The drawing under review shows one solid part. Ordinate dimensions are in mm from its lowest x, y, z. A direction names the side the tool comes from. Give positions to 0.01 mm unless a question says otherwise; leave off trailing zeros. Write each loop counter-clockwise with the first axis right and the second up, starting at its lowest first coordinate (ties: lowest second). Pieces come first, ordered by that corner, then holes. Notation, with made-up numbers: (-7.5, 2) -> (15.5, 2) arc R26 ccw to (15.5, 38) -> close; hole circle Ø4 at (71.25, -35). An arc over 180 degrees is marked (long way). Answer as a JSON object with one key per item and string values.
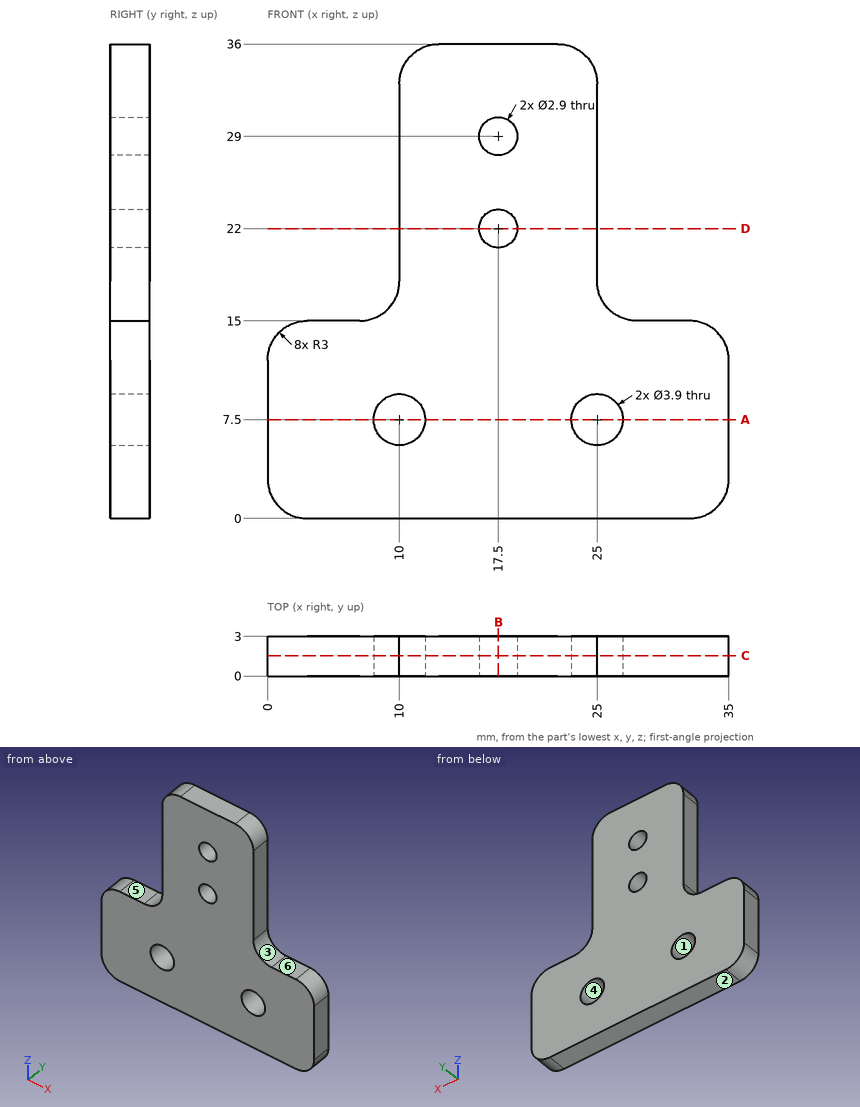
(1) We need section B-B, the plane x = 17.5. State the section outline as (y, z) points.
Here are the results:
{"outline": "(0, 0) -> (3, 0) -> (3, 20.55) -> (0, 20.55) -> close; (0, 23.45) -> (3, 23.45) -> (3, 27.55) -> (0, 27.55) -> close; (0, 30.45) -> (3, 30.45) -> (3, 36) -> (0, 36) -> close"}
(2) Clearance check with flat-ended pins moving along their axes: pin 1 (1.5 mm diameter, centred on x = 30.5, y = 1.5, fed in from +Z); pin 2 (1.5 mm diameter, centred on y = 1, z = 22, fed in from -X); pin 3 (0.9 mm diameter, centred on y = 2, z = 28, fed in from +X); pin 4 (2.5 mm diameter, centred on x = 17.5, z = 22, fed in from -Y). State where each tip first meets the part, or that it passes through.
Here are the results:
{"pin 1": "stops at z = 15", "pin 2": "stops at x = 10", "pin 3": "stops at x = 25", "pin 4": "passes through"}
(3) We need section A-A, the plane z = 7.5. State the section outline as (x, y) points.
Here are the results:
{"outline": "(0, 0) -> (8.05, 0) -> (8.05, 3) -> (0, 3) -> close; (11.95, 0) -> (23.05, 0) -> (23.05, 3) -> (11.95, 3) -> close; (26.95, 0) -> (35, 0) -> (35, 3) -> (26.95, 3) -> close"}
(4) For the marked faces 4, 5 and 6, list the 3-axis set-ups (+Z, -Z, +X, -X, +Y, -Y) from which the entire face can be reached by the end or side of a thin tool; tool diameter is ignored.
Here are the results:
{"face 4": "+Y, -Y", "face 5": "+Z, -X, +Y, -Y", "face 6": "+Z, +X, +Y, -Y"}
(5) The part is to be moulded in two halves that separate along Z. For the marked faces 1, 2 and 3, say which applies: +Z half, -Z half, draft (parallel to the pull), parting line (faces both ways), or undercut.
Here are the results:
{"face 1": "undercut", "face 2": "-Z half", "face 3": "+Z half"}
(6) For line 1 along X through (y, z) = (2.45, 7.5); line 2 along X through (y, z) = (1.85, 29); line 3 along X through (y, z) = (1.6, 30.5), list the stretches that pass through material, from the lowest coordinate up.
Here are the results:
{"line 1": "x = 0 to 8.05, 11.95 to 23.05, 26.95 to 35", "line 2": "x = 10 to 16.05, 18.95 to 25", "line 3": "x = 10 to 25"}
(7) We need section D-D, the plane z = 22. State the section outline as (x, y) points, then the cut area to 3 significant figures.
Here are the results:
{"outline": "(10, 0) -> (16.05, 0) -> (16.05, 3) -> (10, 3) -> close; (18.95, 0) -> (25, 0) -> (25, 3) -> (18.95, 3) -> close", "area": "36.3 mm²"}
(8) We need section C-C, the plane y = 1.55. State the section outline as (x, z) points, then the cut area to 3 significant figures.
Here are the results:
{"outline": "(0, 3) arc R3 ccw to (3, 0) -> (32, 0) arc R3 ccw to (35, 3) -> (35, 12) arc R3 ccw to (32, 15) -> (28, 15) arc R3 cw to (25, 18) -> (25, 33) arc R3 ccw to (22, 36) -> (13, 36) arc R3 ccw to (10, 33) -> (10, 18) arc R3 cw to (7, 15) -> (3, 15) arc R3 ccw to (0, 12) -> close; hole circle Ø3.9 at (10, 7.5); hole circle Ø2.9 at (17.5, 22); hole circle Ø2.9 at (17.5, 29); hole circle Ø3.9 at (25, 7.5)", "area": "795 mm²"}
